The listing builds one solid part. Answer for the finished solid, in the listing's coordinates (mm). A direction names the side the tool comes from. Round coordinates to 2 decimals unless told otherwise and drop trailing zeros. Write each loop counter-clockwise with the first axis right and the second up, starting at its lowest first coordinate (ties: lowest second). Pieces come first, ordered by that corner, then holes.
Item 1: Find section C-C on x = -22. Give the vertices of the cut face in (y, z), then the cut area to 3 significant figures.
Item 2: Find section A-A on x = -36.5. Give the vertices of the cut face in (y, z), then the cut area to 4 significant figures.
Item 3: For a pull along Y with two mould halves and no side action, classify faces 1 (the face through (-34, -5, 0)), 2 (the face through (-60.696, -4.795, 2.218)), 3 (the face through (-1, -8, 2)) as +Y half, -Y half, draft (parallel to the pull), parting line (faces both ways), or undercut.
Item 4: Find section B-B on x = -60. Give the vertices of the cut face in (y, z).
Item 5: Find the intervals of material crossed by probe 1 along X at (y, z) = (-4.5, 3.45); probe 2 along Y at (x, z) = (-5, 3.55) (3 decimals); probe 3 along Y at (x, z) = (-55, 3.35), in increasing order.
Item 6: A tool of negligible diameter and unlimited length cuts with its end or side. For faces 4 (the face through (-65.945, -1.752, 2.219)), 5 (the face through (-26, 0, 2)), 6 (the face through (-46.35, -5.06, 2.22)), 7 (the face through (-54.9, 4.7, 2.2)), 8 (the face through (-26, -10, 2)), from which of +Z, -Z, +X, -X, +Y, -Y can it reach the whole face along a straight path? Write none if from no direction.
Item 7: Each of these flat-tipped pins is pushed along its axis until it touches: pin 1 (3 mm diameter, centred on x = -63.5, y = -5, fed in from +Z); pin 2 (5 mm diameter, centred on x = -49, y = -5, fed in from +Z); pin 3 (2 mm diameter, centred on x = -10.5, z = 2.5, fed in from -Y). Where does it stop, or does it pass through?
Item 8: Find section D-D on z = 3.3. Give the number of separate pieces and of enclosed holes in the cut face, then the cut area to 3 significant figures.
```python
from build123d import *

# Parameters (mm, degrees)
SKETCH_1_R      = 1.025
SKETCH_1_R_2    = 1.25
EXTRUDE_1_DEPTH = 4.5
FILLET_1_R      = 1
FILLET_2_R      = 5
FILLET_3_R      = 5


# Some blends are built 0.0001 mm under size
with BuildPart() as part:
    # 草图1 → 凸台-拉伸1 (new body)
    with BuildSketch(Plane.XY):
        with BuildLine():
            Line((-63.312039461, 0), (-67, 0))
            Line((-67, 0), (-67, -10))
            Line((-67, -10), (-63.312039461, -10))
            ThreePointArc((-63.312039461, -10), (-55, -14.7), (-46.687960539, -10))
            Line((-46.687960539, -10), (0, -10))
            Line((0, -10), (0, 0))
            Line((0, 0), (-46.687960539, 0))
            ThreePointArc((-46.687960539, 0), (-55, 4.7), (-63.312039461, 0))
        make_face()
        with Locations((-5, -5)):
            Circle(SKETCH_1_R, mode=Mode.SUBTRACT)
        with Locations((-63.5, -5)):
            Circle(SKETCH_1_R_2, mode=Mode.SUBTRACT)
        with Locations((-36.5, -5)):
            Circle(SKETCH_1_R_2, mode=Mode.SUBTRACT)
        with BuildLine():
            ThreePointArc((-49.877708333, -2.49957442), (-60.7, -5), (-49.877708333, -7.50042558))
            ThreePointArc((-49.877708333, -7.50042558), (-46.35, -5), (-49.877708333, -2.49957442))
        make_face(mode=Mode.SUBTRACT)
    extrude(amount=EXTRUDE_1_DEPTH)

    # 圆角1
    fillet_1_edges = [part.edges().sort_by_distance(p)[0] for p in [
        (-49.877708333, -7.50042558, 2.25),
        (-49.877708333, -2.49957442, 2.25),
    ]]
    fillet(fillet_1_edges, radius=FILLET_1_R)

    # 圆角2
    fillet_2_edges = [part.edges().sort_by_distance(p)[0] for p in [
        (0, -10, 2.25),
        (0, 0, 2.25),
    ]]
    fillet(fillet_2_edges, radius=FILLET_2_R - 0.0001)  # a hair under: the kernel refuses the full size

    # 圆角3
    # the kernel refuses this fillet: 5 mm, written as the material it takes off along each edge
    with BuildSketch(Plane(origin=(-67, 0, -12.061963059), x_dir=(0, -1, 0), z_dir=(0, 0, 1))) as fillet_3_piece_1:
        with BuildLine():
            CenterArc((4.824785224, 5), FILLET_3_R, 195.212986046, 74.787013954)
            Line((0, 3.687960539), (-0.096495704, 3.66171975))
            ThreePointArc((-0.096495704, 3.66171975), (-0.1, 1.84398027), (-0.1, 0))
            Line((-0.1, 0), (0, -0.1))
            Line((0, -0.1), (4.824785224, -0.1))
            Line((4.824785224, -0.1), (4.824785224, 0))
        make_face()
    extrude(amount=28.623926118, mode=Mode.SUBTRACT)
    with BuildSketch(Plane(origin=(-67, -10, -12.061963059), x_dir=(1, 0, 0), z_dir=(0, 0, 1))) as fillet_3_piece_2:
        with BuildLine():
            CenterArc((5, 4.824785224), FILLET_3_R, 180, 74.787013954)
            Line((0, 4.824785224), (-0.1, 4.824785224))
            Line((-0.1, 4.824785224), (-0.1, 0))
            Line((-0.1, 0), (0, -0.1))
            ThreePointArc((0, -0.1), (1.84398027, -0.1), (3.66171975, -0.096495704))
            Line((3.66171975, -0.096495704), (3.687960539, 0))
        make_face()
    extrude(amount=28.623926118, mode=Mode.SUBTRACT)


solid = part.part
```
Check values:
1. outline: (-10, 0) - (0, 0) - (0, 4.5) - (-10, 4.5) - close
1. area: 45.0 mm2
2. outline: (-10, 0) - (-6.25, 0) - (-6.25, 4.5) - (-10, 4.5) - close; (-3.75, 0) - (0, 0) - (0, 4.5) - (-3.75, 4.5) - close
2. area: 33.75 mm2
3. face 1: draft
3. face 2: undercut
3. face 3: -Y half
4. outline: (-13.31, 0) - (-7.74, 0) - (-7.74, 4.5) - (-13.31, 4.5) - close; (-2.26, 0) - (3.31, 0) - (3.31, 4.5) - (-2.26, 4.5) - close
5. probe 1: x = -66.99 to -64.65, -62.35 to -60.68, -46.4 to -37.65, -35.35 to -5.89, -4.11 to -0.03
5. probe 2: y = -10 to -6.025, -3.975 to 0
5. probe 3: y = -14.7 to -10.7, 0.7 to 4.7
6. face 4: +Z, -Z, -X, +Y
6. face 5: +Z, -Z, +X, +Y
6. face 6: +Z, -Z
6. face 7: +Z, -Z, +Y
6. face 8: +Z, -Z, +X, -Y
7. pin 1: stops at z = 4.5
7. pin 2: passes through
7. pin 3: stops at y = -10
8. separate pieces: 1
8. enclosed holes: 4
8. area: 632 mm2
